```python
from build123d import *

# Parameters (mm, degrees)
SKETCH1_R             = 18
BOSS_EXTRUDE1_DEPTH   = 2
F_2_0MM_DOWEL_HOLE1_D = 2
SKETCH5_R             = 1.6
CUT_EXTRUDE4_DEPTH    = 42.060930335


with BuildPart() as part:
    # Sketch1 → Boss-Extrude1 (new body)
    with BuildSketch(Plane.XY):
        with BuildLine():
            ThreePointArc((-29, 0), (0, -29), (29, 0))
            ThreePointArc((29, 0), (0, 29), (-29, 0))
        make_face()
        Circle(SKETCH1_R, mode=Mode.SUBTRACT)
    extrude(amount=BOSS_EXTRUDE1_DEPTH)

    # Ø2.0mm Dowel Hole1 (through all)
    with Locations(Plane(origin=(-19, 19, 2), x_dir=(1, 0, 0), z_dir=(0, 0, 1))):
        with Locations((0, 0), (2, -2), (36, -2), (38, 0), (36, -36), (38, -38), (0, -38), (2, -36)):
            Hole(F_2_0MM_DOWEL_HOLE1_D / 2)

    # Sketch5 → Cut-Extrude4 (cut, through all)
    with BuildSketch(Plane.XY):
        with Locations((0, 25)):
            Circle(SKETCH5_R)
        with Locations((-25, 0)):
            Circle(SKETCH5_R)
        with Locations((25, 0)):
            Circle(SKETCH5_R)
        with Locations((0, -25)):
            Circle(SKETCH5_R)
    extrude(amount=CUT_EXTRUDE4_DEPTH, mode=Mode.SUBTRACT)


solid = part.part
```
Source: CAD feature listing. Evaluate the final solid. Frame: model axes, mm. Round coordinates to 2 decimals unless told otherwise and drop trailing zeros. Write each loop counter-clockwise with the first axis right and the second up, starting at its lowest first coordinate (ties: lowest second). Pieces come first, ordered by that corner, then holes. Notation, with made-up numbers: M -25,-12.5 L -14,-12.5 A36 cw -14,22.5 Z; hole C 5,-31 d9. An arc over 180 degrees is marked long. Answer as a JSON object with one key per item and string values. Group by question number.
(1) Section query A-A on y = 0. Output: boundary loops of the cut face in (x, z).
(2) Section query C-C on x = 15. Output: boundary loops of the cut face in (y, z), then the cut area to 3 significant figures.
(3) Section query B-B on z = 1.3. State how many separate pieces and enclosed holes the cut face has, then the cut area to 3 significant figures.
(4) Section query D-D on x = -19. Output: boundary loops of the cut face in (y, z), then the cut area to 3 significant figures.
(5) Mould query, pull axis X, two halves, no side actions, for faces 1 (the cylindrical face through (-0.208, -23.414, 0.986)), 2 (the cylindrical face through (26.789, -11.107, 0.986)), 3 (the flat face through (-13.3, -12.5, 2)). Classes: +X half, -X half, draft (parallel to the pull), parting line (faces both ways), or undercut.
(6) First-contact query: pin 1 (1.6 mm diameter, centred on x = 19, y = 19, fed in from -Z). Flat tip, straight axial feed; report the tip coordinate or a pass-through.
(7) Ray query, line 1 (Y direction, x = 0, z = 0.95); line 2 (Y direction, x = 18.5, z = 0.15); line 3 (Y direction, x = -3, z = 0.4). Return the intervals inside material, ascending. Write a range as [from, to].
Computed values:
{
 "1": {"outline": "M -29,0 L -26.6,0 L -26.6,2 L -29,2 Z; M -23.4,0 L -18,0 L -18,2 L -23.4,2 Z; M 18,0 L 23.4,0 L 23.4,2 L 18,2 Z; M 26.6,0 L 29,0 L 29,2 L 26.6,2 Z"},
 "2": {"outline": "M -24.82,0 L -9.95,0 L -9.95,2 L -24.82,2 Z; M 9.95,0 L 24.82,0 L 24.82,2 L 9.95,2 Z", "area": "59.5 mm^2"},
 "3": {"separate pieces": "1", "enclosed holes": "13", "area": "1,570 mm^2"},
 "4": {"outline": "M -21.91,0 L -20,0 L -20,2 L -21.91,2 Z; M -18,0 L 18,0 L 18,2 L -18,2 Z; M 20,0 L 21.91,0 L 21.91,2 L 20,2 Z", "area": "79.6 mm^2"},
 "5": {"face 1": "undercut", "face 2": "parting line", "face 3": "draft"},
 "6": {"pin 1": "through"},
 "7": {"line 1": "[-29, -26.6], [-23.4, -18], [18, 23.4], [26.6, 29]", "line 2": "[-22.33, -19.87], [-18.13, 18.13], [19.87, 22.33]", "line 3": "[-28.84, -17.75], [17.75, 28.84]"}
}
